Model file for the job. Use its own axes, mm. Give positions to 0.01 mm unless a question says otherwise; leave off trailing zeros. Order: outer loops, then holes, each group sorted by start corner. A loop starts at its lowest first (then second) coordinate and runs counter-clockwise, first axis right, second up. Notation, with made-up numbers: (28.25, 0) -> (80.25, 0) arc R21 ccw to (80.25, 35) -> close; hole circle Ø4 at (-23.5, -27). An arc over 180 degrees is marked (long way). Use CSV: the item, a comma, the result in double quotes. Start each with the question number.
1. Drop flat-ended pins along their axis: pin 1 (5 mm diameter, centred on x = -7, y = 8.5, fed in from -Z); pin 2 (16.5 mm diameter, centred on x = 0, z = 0, fed in from -Y); pin 3 (12 mm diameter, centred on y = 5.5, z = 0.5, fed in from -X); pin 4 (6 mm diameter, centred on y = 8, z = 2, fed in from +X). Give the stop position or say it passes through.
2. Wall check: line 1 (X direction, y = -4, z = 0); line 2 (X direction, y = 0.5, z = 5.5). Give the ranges that are in metal, low to high. Write a range as from..to.
3. Cut at A-A on x = 0. List the corners of the cut face in (y, z).
4. Cut at D-D on y = 0.75. List the corners of the cut face in (x, z), then the cut area to 3 significant figures.
5. Cut at C-C on y = -4.5. List the corners of the cut face in (x, z), then the cut area to 3 significant figures.
6. Cut at B-B on z = 0. List the corners of the cut face in (x, y), then the cut area to 3 significant figures.
7. Pull direction X, two halves, no side cores. Call faces 1 (the flat face through (6, -10, -13)), 2 (the cylindrical face through (-13.64, -4.93, 10.46)), 3 (the cylindrical face through (13.26, -4.93, -4.18)), 4 (the conical face through (-1.63, 14.3, -7.36)): released by +X, released by -X, zero draft, split by the parting line, or undercut.
Autodesk Inventor part; units mm, degrees
ref_plane "YZ Plane" through (0, 0, 0) normal (1, 0, 0) x (0, 1, 0)
ref_plane "XZ Plane" through (0, 0, 0) normal (0, 1, 0) x (-1, 0, 0)
ref_plane "XY Plane" through (0, 0, 0) normal (0, 0, 1) x (1, 0, 0)
sketch "Boceto2" plane through (0, 0, 0) normal (0, 0, 1) x (1, 0, 0)
  line L0 (0, 0) -> (0, 20)
  dimension "d2" = 20
ref_plane "Plano de trabajo1" through (0, 20, 0) normal (0, 1, 0) x (-1, 0, 0)
sketch "Boceto4" plane through (0, 20, 0) normal (0, 1, 0) x (-1, 0, 0)
  circle A0 centre (0, 0) radius 5
  circle A1 centre (0, 0) radius 7
  dimension "d13" = 10
  dimension "d14" = 14
extrude "Extrusión1" add sketch "Boceto4" against normal blind 20 draft 27
sketch "Boceto7" plane through (0, 20, 0) normal (0, 1, 0) x (1, 0, 0)
  circle A0 centre (0, 0) radius 7
  circle A1 centre (0, 0) radius 5
extrude "Extrusión2" cut sketch "Boceto7" against normal blind 20 draft 24 contours A1
sketch "Boceto9" plane through (0, 0, 0) normal (0, -1, 0) x (1, 0, 0)
  circle A0 centre (0, 0) radius 13.9046
  circle A1 centre (0, 0) radius 13.9046
  circle A2 centre (0, 0) radius 17.1905
extrude "Extrusión3" add sketch "Boceto9" along normal blind 10
properties part number "Boquilla"
Verdict:
1,pin 1,"z = -12.74"
1,pin 2,"y = 12.7"
1,pin 3,"x = -17.19"
1,pin 4,"x = 14.54"
2,line 1,"-17.19..-13.9, 13.9..17.19"
2,line 2,"-16.02..-12.53, 12.53..16.02"
3,outline,"(-10, -17.19) -> (0, -17.19) -> (20, -7) -> (20, -5) -> (0, -13.9) -> (-10, -13.9) -> close; (-10, 13.9) -> (0, 13.9) -> (20, 5) -> (20, 7) -> (0, 17.19) -> (-10, 17.19) -> close"
4,outline,"circle Ø33.62 at (0, 0); hole circle Ø27.14 at (0, 0)"
4,area,"309 mm^2"
5,outline,"circle Ø34.38 at (0, 0); hole circle Ø27.81 at (0, 0)"
5,area,"321 mm^2"
6,outline,"(-17.19, -10) -> (-13.9, -10) -> (-13.9, 0) -> (-5, 20) -> (-7, 20) -> (-17.19, 0) -> close; (5, 20) -> (13.9, 0) -> (13.9, -10) -> (17.19, -10) -> (17.19, 0) -> (7, 20) -> close"
6,area,"171 mm^2"
7,face 1,"zero draft"
7,face 2,"split by the parting line"
7,face 3,"undercut"
7,face 4,"undercut"
